Here's how the part is built. I have some questions about the finished solid (model axes, mm). A direction names the side the tool comes from. Give positions to 0.01 mm unless a question says otherwise; leave off trailing zeros. Order: outer loops, then holes, each group sorted by start corner. A loop starts at its lowest first (then second) coordinate and runs counter-clockwise, first axis right, second up. Notation, with made-up numbers: (-16.5, -30) - (10.5, -30) arc R26 ccw to (10.5, 7) - close; hole circle Ø10 at (74.25, -38). An arc over 180 degrees is marked (long way). One line per question, with ' | ' between items.
from build123d import *

# Parameters (mm, degrees)
SKETCH1_R               = 5
BOSS_EXTRUDE1_DEPTH     = 67.5
CUT_EXTRUDE1_DEPTH      = 68.869359802
CUT_EXTRUDE1_DEPTH_BACK = 68.869359802
SKETCH2_W               = 4
SKETCH2_H               = 24
CUT_EXTRUDE2_DEPTH      = 68.869359802
CUT_EXTRUDE2_DEPTH_BACK = 68.869359802
SKETCH3_R               = 1.55


with BuildPart() as part:
    # Sketch1 → Boss-Extrude1 (new, symmetric)
    with BuildSketch(Plane(origin=(0, 0, 0), x_dir=(1, 0, 0), z_dir=(0, 1, 0))):
        with Locations(Location((0, 0, 0), (0, 0, 270))):
            Circle(SKETCH1_R)
    extrude(amount=BOSS_EXTRUDE1_DEPTH, both=True)

    # Sketch2 → Cut-Extrude1 (cut, two sides: drawn at the far end of the back side and taken through both)
    with BuildSketch(Plane.XY.offset(-CUT_EXTRUDE1_DEPTH_BACK)):
        with Locations((0, -55.5)):
            Rectangle(SKETCH2_W, SKETCH2_H)
    extrude(amount=CUT_EXTRUDE1_DEPTH + CUT_EXTRUDE1_DEPTH_BACK, mode=Mode.SUBTRACT)

    # Sketch3 → Cut-Extrude2 (cut, two sides: drawn at the far end of the back side and taken through both)
    with BuildSketch(Plane(origin=(0, 0, 0), x_dir=(0, 0, -1), z_dir=(1, 0, 0)).offset(-CUT_EXTRUDE2_DEPTH_BACK)):
        with Locations((0, -63.5)):
            Circle(SKETCH3_R)
    extrude(amount=CUT_EXTRUDE2_DEPTH + CUT_EXTRUDE2_DEPTH_BACK, mode=Mode.SUBTRACT)


solid = part.part
1) Please list where these lines run through material, in increasing order: L1, parallel to Y at x = 3.6, z = 0; L2, parallel to Y at x = 0.25, z = -2.5; L3, parallel to Z at x = 2.65, y = -63.5.
Model answer:
L1: y = -67.5 to -65.05, -61.95 to 67.5 | L2: y = -43.5 to 67.5 | L3: z = -4.24 to -1.55, 1.55 to 4.24
2) I'm going to push flat-ended pins straight in: P1, Ø1.5, axis at y = -24, z = -3.5, coming from the +X side; P2, Ø1.9, axis at y = -63.5, z = 0, coming from the +X side; P3, Ø1, axis at x = 3.5, y = -8.5, coming from the -Z side; P4, Ø2, axis at x = -0.5, z = 2, coming from the -Y side. Where does each tip first touch, or does it pass through?
Model answer:
P1: stops at x = 4.18 | P2: passes through | P3: stops at z = -4 | P4: stops at y = -43.5
3) I want a section at C-C (x = 0). List the corners of the cut face in (y, z) for me, plus the area to 3 significant figures.
Model answer:
outline: (-43.5, -5) - (67.5, -5) - (67.5, 5) - (-43.5, 5) - close | area: 1,110 mm2
4) Thinking about a two-plate mould opening in X: for faces 1 (the face through (0, 1, -5)), 2 (the face through (2, -56, 0)), 3 (the face through (3.48, -63.43, 1.55)), which applies, +X half, -X half, draft (parallel to the pull), parting line (faces both ways), or undercut?
Model answer:
face 1: parting line | face 2: undercut | face 3: draft
5) I want a section at D-D (y = 44). List the corners of the cut face in (x, z) for me.
Model answer:
outline: circle Ø10 at (0, 0)
6) I want a section at A-A (z = 0). List the corners of the cut face in (x, y) for me, plus the area to 3 significant figures.
Model answer:
outline: (-5, -67.5) - (-2, -67.5) - (-2, -65.05) - (-5, -65.05) - close; (-5, -61.95) - (-2, -61.95) - (-2, -43.5) - (2, -43.5) - (2, -61.95) - (5, -61.95) - (5, 67.5) - (-5, 67.5) - close; (2, -67.5) - (5, -67.5) - (5, -65.05) - (2, -65.05) - close | area: 1,240 mm2
7) On a 3-axis mill with a long thin cutter (end or side, diameter ignored), from which of +Z, -Z, +X, -X, +Y, -Y can I reach the whole of each face in a straight line? I mean faces 4 (the face through (-3, -67.5, 0)), 5 (the face through (0, -43.5, 0)). Say none if no direction works.
Model answer:
face 4: +Z, -Z, +X, -X, -Y | face 5: +Z, -Z, -Y
8) I want a section at B-B (y = -63.5). List the corners of the cut face in (x, z) for me.
Model answer:
outline: (-4.75, -1.55) arc R5 ccw to (-2, -4.58) - (-2, -1.55) - close; (-4.75, 1.55) - (-2, 1.55) - (-2, 4.58) arc R5 ccw to start; (2, -4.58) arc R5 ccw to (4.75, -1.55) - (2, -1.55) - close; (2, 1.55) - (4.75, 1.55) arc R5 ccw to (2, 4.58) - close
